Can you work these out from the model? Positions are in its coordinate system, mm. Face numbers are marked on the shaded views. A direction names the side the tool comes from. Give positions to 0.01 mm unless a question says otherwise; leave off trailing zeros. Write each loop counter-clockwise with the first axis right and the second up, starting at its lowest first coordinate (ties: lowest second). Pieces come first, ordered by that corner, then holes. Notation, with made-up numbers: (8.5, -35) -> (42.5, -35) arc R29 cw to (42.5, -6) -> close; hole circle Ø6 at (46.25, 43). An arc over 180 degrees is marked (long way). One line per item, written item: value.
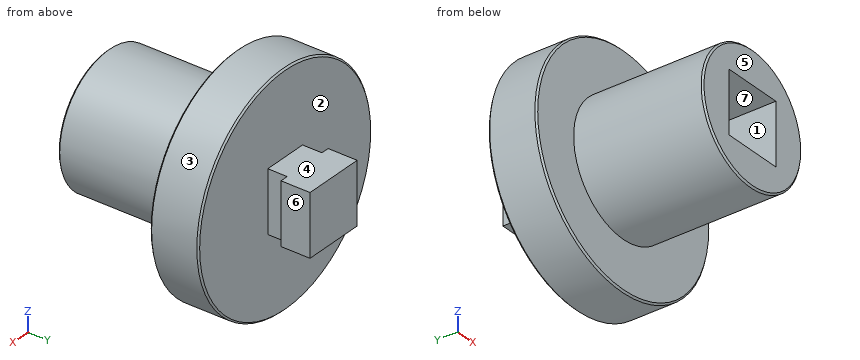
from build123d import *

# Parameters (mm, degrees)
SKETCH1_R           = 4
BOSS_EXTRUDE1_DEPTH = 11
SKETCH2_W           = 3.8
SKETCH2_H           = 3.8
CUT_EXTRUDE1_DEPTH  = 4
SKETCH3_W           = 3.8
SKETCH3_H           = 3.8
BOSS_EXTRUDE2_DEPTH = 3
SKETCH4_W           = 0.5
SKETCH4_H           = 1.2
CUT_EXTRUDE2_DEPTH  = 13
SKETCH5_R           = 7
BOSS_EXTRUDE3_DEPTH = 3
CHAMFER1_SIZE       = 0.1


with BuildPart() as part:
    # Sketch1 → Boss-Extrude1 (new body)
    with BuildSketch(Plane(origin=(0, 0, 0), x_dir=(1, 0, 0), z_dir=(0, 1, 0))):
        Circle(SKETCH1_R)
    extrude(amount=BOSS_EXTRUDE1_DEPTH)

    # Sketch2 → Cut-Extrude1 (cut)
    with BuildSketch(Plane.XZ):
        Rectangle(SKETCH2_W, SKETCH2_H)
    extrude(amount=-CUT_EXTRUDE1_DEPTH, mode=Mode.SUBTRACT)

    # Sketch3 → Boss-Extrude2 (add)
    with BuildSketch(Plane(origin=(0, 11, 0), x_dir=(1, 0, 0), z_dir=(0, 1, 0))):
        Rectangle(SKETCH3_W, SKETCH3_H)
    extrude(amount=BOSS_EXTRUDE2_DEPTH)

    # Sketch4 → Cut-Extrude2 (cut)
    with BuildSketch(Plane.XY.offset(1.9)):
        with Locations((-1.65, 11.6)):
            Rectangle(SKETCH4_W, SKETCH4_H)
        with Locations((1.65, 11.6)):
            Rectangle(SKETCH4_W, SKETCH4_H)
    extrude(amount=-CUT_EXTRUDE2_DEPTH, mode=Mode.SUBTRACT)

    # Sketch5 → Boss-Extrude3 (add)
    with BuildSketch(Plane(origin=(0, 11, 0), x_dir=(1, 0, 0), z_dir=(0, 1, 0))):
        Circle(SKETCH5_R)
    extrude(amount=-BOSS_EXTRUDE3_DEPTH)

    # Chamfer1
    chamfer1_edges = [part.edges().sort_by_distance(p)[0] for p in [
        (-4, 0, 0),
        (-7, 11, 0),
        (-7, 8, 0),
    ]]
    chamfer(chamfer1_edges, length=CHAMFER1_SIZE)


solid = part.part
1) If we section it at C-C (y = 5.5): Write out the boundary of the cut face in (x, z), and give its area (3 significant figures).
Answer list:
outline: circle Ø8 at (0, 0)
area: 50.3 mm^2
2) We'd pull the mould along Z, two halves only. Please class the marked faces 1, 2, 3 and 4: released by +Z, released by -Z, zero draft, split by the parting line, or undercut.
Answer list:
face 1: undercut
face 2: zero draft
face 3: split by the parting line
face 4: released by +Z
3) I need wall thicknesses on L1, parallel to Y at x = 0.75, z = -3; L2, parallel to Z at x = -0.75, y = 2.5; L3, parallel to Y at x = 3, z = 4. Which ranges of each line are inside material? Lowest first, please.
Answer list:
L1: y = 0 to 11
L2: z = -3.93 to -1.9, 1.9 to 3.93
L3: y = 8 to 11
4) If we section it at B-B (z = 0): Write out the boundary of the cut face in (x, y), and give its area (3 significant figures).
Answer list:
outline: (-7, 8.1) -> (-6.9, 8) -> (-4, 8) -> (-4, 0.1) -> (-3.9, 0) -> (-1.9, 0) -> (-1.9, 4) -> (1.9, 4) -> (1.9, 0) -> (3.9, 0) -> (4, 0.1) -> (4, 8) -> (6.9, 8) -> (7, 8.1) -> (7, 10.9) -> (6.9, 11) -> (1.4, 11) -> (1.4, 12.2) -> (1.9, 12.2) -> (1.9, 14) -> (-1.9, 14) -> (-1.9, 12.2) -> (-1.4, 12.2) -> (-1.4, 11) -> (-6.9, 11) -> (-7, 10.9) -> close
area: 101 mm^2
5) If we section it at A-A (x = 0): Write out the boundary of the cut face in (y, z).
Answer list:
outline: (0, -3.9) -> (0.1, -4) -> (8, -4) -> (8, -6.9) -> (8.1, -7) -> (10.9, -7) -> (11, -6.9) -> (11, -1.9) -> (14, -1.9) -> (14, 1.9) -> (11, 1.9) -> (11, 6.9) -> (10.9, 7) -> (8.1, 7) -> (8, 6.9) -> (8, 4) -> (0.1, 4) -> (0, 3.9) -> (0, 1.9) -> (4, 1.9) -> (4, -1.9) -> (0, -1.9) -> close
6) For the marked faces 5, 6 and 7, which set-ups out of +Z, -Z, +X, -X, +Y, -Y let a thin tool reach every point of the face, with its end or its side?
Answer list:
face 5: +Z, -Z, +X, -X, -Y
face 6: +Z, -Z, +X, +Y
face 7: -Y
7) Will these pins go through, and if not, where does the flat tip stop? pin 1 (0.5 mm diameter, centred on y = 13, z = 0.5, fed in from +X); pin 2 (3 mm diameter, centred on x = 0, y = 1, fed in from +Z); pin 3 (0.6 mm diameter, centred on y = 11.5, z = 0.5, fed in from +X); pin 4 (7 mm diameter, centred on x = -2.5, z = 2.5, fed in from -Y).
Answer list:
pin 1: stops at x = 1.9
pin 2: stops at z = 4
pin 3: stops at x = 1.4
pin 4: stops at y = 0
